Autodesk Inventor part; units mm, degrees
ref_plane "YZ Plane" through (0, 0, 0) normal (1, 0, 0) x (0, 1, 0)
ref_plane "XZ Plane" through (0, 0, 0) normal (0, 1, 0) x (-1, 0, 0)
ref_plane "XY Plane" through (0, 0, 0) normal (0, 0, 1) x (1, 0, 0)
sketch "Sketch1" plane through (0, 0, 0) normal (0, 0, 1) x (1, 0, 0)
  circle A0 centre (0, 0) radius 2
  circle A1 centre (0, 0) radius 7
  circle A2 centre (0, 0) radius 3 construction
  circle A3 centre (0, 0) radius 5.5 construction
  line L0 (2.9047, 0.75) -> (5.2915, 1.5)
  line L1 (2.9047, -0.75) -> (5.2915, -1.5)
  arc A4 (2.9047, -0.75) -> (2.9047, 0.75) centre (0, 0) ccw
  arc A5 (5.2915, -1.5) -> (5.2915, 1.5) centre (0, 0) ccw
  line L2 (0, 0) -> (8.9421, 0) construction
  circle A6 centre (0, 0) radius 3 construction
  circle A7 centre (0, 0) radius 5.5 construction
  line L3 (0.8028, 2.8906) -> (1.3467, 5.3326)
  line L4 (2.1019, 2.1406) -> (3.9448, 3.8326)
  arc A8 (2.1019, 2.1406) -> (0.8028, 2.8906) centre (0, 0) ccw
  arc A9 (3.9448, 3.8326) -> (1.3467, 5.3326) centre (0, 0) ccw
  line L5 (0, 0) -> (4.471, 7.7441) construction
  circle A10 centre (0, 0) radius 3 construction
  circle A11 centre (0, 0) radius 5.5 construction
  line L6 (-2.1019, 2.1406) -> (-3.9448, 3.8326)
  line L7 (-0.8028, 2.8906) -> (-1.3467, 5.3326)
  arc A12 (-0.8028, 2.8906) -> (-2.1019, 2.1406) centre (0, 0) ccw
  arc A13 (-1.3467, 5.3326) -> (-3.9448, 3.8326) centre (0, 0) ccw
  line L8 (0, 0) -> (-4.471, 7.7441) construction
  circle A14 centre (0, 0) radius 3 construction
  circle A15 centre (0, 0) radius 5.5 construction
  line L9 (-2.9047, -0.75) -> (-5.2915, -1.5)
  line L10 (-2.9047, 0.75) -> (-5.2915, 1.5)
  arc A16 (-2.9047, 0.75) -> (-2.9047, -0.75) centre (0, 0) ccw
  arc A17 (-5.2915, 1.5) -> (-5.2915, -1.5) centre (0, 0) ccw
  line L11 (0, 0) -> (-8.9421, 0) construction
  circle A18 centre (0, 0) radius 3 construction
  circle A19 centre (0, 0) radius 5.5 construction
  line L12 (-0.8028, -2.8906) -> (-1.3467, -5.3326)
  line L13 (-2.1019, -2.1406) -> (-3.9448, -3.8326)
  arc A20 (-2.1019, -2.1406) -> (-0.8028, -2.8906) centre (0, 0) ccw
  arc A21 (-3.9448, -3.8326) -> (-1.3467, -5.3326) centre (0, 0) ccw
  line L14 (0, 0) -> (-4.471, -7.7441) construction
  circle A22 centre (0, 0) radius 3 construction
  circle A23 centre (0, 0) radius 5.5 construction
  line L15 (2.1019, -2.1406) -> (3.9448, -3.8326)
  line L16 (0.8028, -2.8906) -> (1.3467, -5.3326)
  arc A24 (0.8028, -2.8906) -> (2.1019, -2.1406) centre (0, 0) ccw
  arc A25 (1.3467, -5.3326) -> (3.9448, -3.8326) centre (0, 0) ccw
  line L17 (0, 0) -> (4.471, -7.7441) construction
  dimension "d0" = 4
  dimension "d1" = 14
  dimension "d2" = 6
  dimension "d3" = 11
  dimension "d4" = 0.75
  dimension "d5" = 0.75
  dimension "d8" = 360
extrude "Extrusion1" add sketch "Sketch1" along normal blind 5
fillet "Fillet1" radius 2.25 2 edges at (-7, 0, 5) (-7, 0, 0)
properties part number "Wheel" material "ABS Plastic"
CAD build for the part. Positions are in the model's coordinates, mm. Coordinates: 2 decimals unless noted, no trailing zeros. Loops run counter-clockwise (first coordinate to the right, second up) from the corner with the lowest first, then second, coordinate; pieces in that order, holes last. Notation, with made-up numbers: (36.25, 80) - (56.25, 80) arc R25 ccw to (56.25, 108) - close; hole circle Ø11 at (-28.5, 58.25). An arc over 180 degrees is marked (long way). Use CSV: the item, a comma, the result in double quotes. Start each with the question number.
Q1. Cut at C-C, the plane z = 1.55. List the corners of the cut face in (x, y).
Q2. Cut at A-A, the plane y = 0. List the corners of the cut face in (x, z).
Q3. Cut at D-D, the plane y = 2.5. State how many separate pieces and enclosed holes the cut face has, then the cut area to 3 significant figures.
Q4. Cut at B-B, the plane x = 0. List the corners of the cut face in (y, z), then the cut area to 3 significant figures.
Q5. Probe probe 1 along Y at (x, z) = (0, 2.2); probe 2 along Y at (x, z) = (-1.5, 0.9); probe 3 along X at (y, z) = (3.75, 1.8). List the from-to ranges inside material, lowest first. Write a range as from..to.
Q6. Drop a flat-ended pin along its axis: P1, Ø1, axis at y = -2, z = 1.5, coming from the +X side. Give the stop position or say it passes through.
Here are the results:
1,outline,"circle Ø13.78 at (0, 0); hole (-5.29, -1.5) - (-2.9, -0.75) arc R3 cw to (-2.9, 0.75) - (-5.29, 1.5) arc R5.5 ccw to start; hole (-3.94, -3.83) arc R5.5 ccw to (-1.35, -5.33) - (-0.8, -2.89) arc R3 cw to (-2.1, -2.14) - close; hole (-3.94, 3.83) - (-2.1, 2.14) arc R3 cw to (-0.8, 2.89) - (-1.35, 5.33) arc R5.5 ccw to start; hole circle Ø4 at (0, 0); hole (0.8, -2.89) - (1.35, -5.33) arc R5.5 ccw to (3.94, -3.83) - (2.1, -2.14) arc R3 cw to start; hole (0.8, 2.89) arc R3 cw to (2.1, 2.14) - (3.94, 3.83) arc R5.5 ccw to (1.35, 5.33) - close; hole (2.9, -0.75) - (5.29, -1.5) arc R5.5 ccw to (5.29, 1.5) - (2.9, 0.75) arc R3 cw to start"
2,outline,"(-7, 2.25) arc R2.25 ccw to (-5.5, 0.13) - (-5.5, 4.87) arc R2.25 ccw to (-7, 2.75) - close; (-3, 0) - (-2, 0) - (-2, 5) - (-3, 5) - close; (2, 0) - (3, 0) - (3, 5) - (2, 5) - close; (5.5, 0.13) arc R2.25 ccw to (7, 2.25) - (7, 2.75) arc R2.25 ccw to (5.5, 4.87) - close"
3,separate pieces,"3"
3,enclosed holes,"0"
3,area,"52.3 mm2"
4,outline,"(-7, 2.25) arc R2.25 ccw to (-4.75, 0) - (-2, 0) - (-2, 5) - (-4.75, 5) arc R2.25 ccw to (-7, 2.75) - close; (2, 0) - (4.75, 0) arc R2.25 ccw to (7, 2.25) - (7, 2.75) arc R2.25 ccw to (4.75, 5) - (2, 5) - close"
4,area,"45.7 mm2"
5,probe 1,"-7..-2, 2..7"
5,probe 2,"-6.38..-5.29, -2.6..-1.32, 1.32..2.6, 5.29..6.38"
5,probe 3,"-5.86..-3.85, -0.99..0.99, 3.85..5.86"
6,P1,"x = 6.77"
